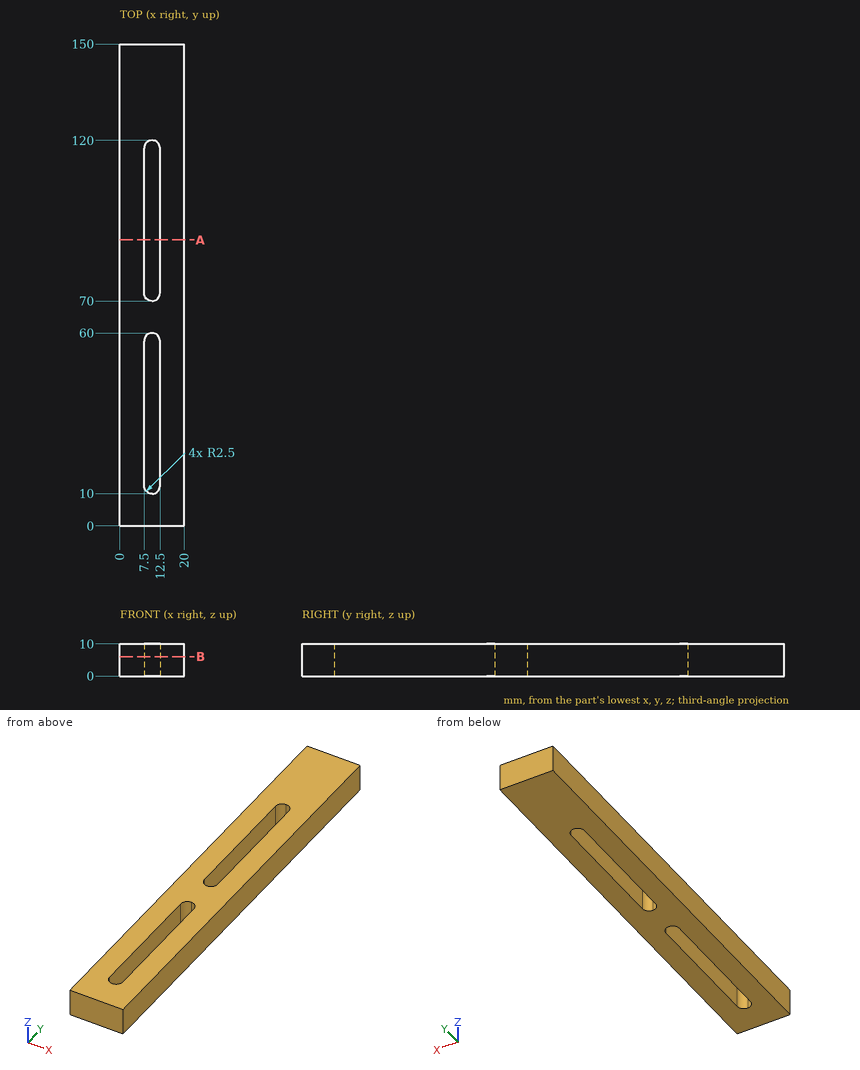
Geometry check sheet. Reference: drawing and pictorial views, mm from the part's lowest x, y, z. Give positions to 0.01 mm unless a question says otherwise; leave off trailing zeros. Write each loop counter-clockwise with the first axis right and the second up, starting at its lowest first coordinate (ties: lowest second). Pieces come first, ordered by that corner, then holes. Notation, with made-up numbers: M 21,22.25 L 54,22.25 A14 cw 54,30.25 Z; hole C 75,37 d1. An arc over 180 degrees is marked long. Put each result on its own line as item: value. Start each with the question number.
1. Scan line: line 1 along X through (y, z) = (72.5, 7). Record every from-to range of solid material in increasing order. Write a range as [from, to].
2. Section check A-A (y = 89). Record the cut outline in (x, z), and give its area (3 significant figures).
3. Section check B-B (z = 6). Give the number of separate pieces and of enclosed holes in the cut face, and give its area (3 significant figures).
Answer list:
1. line 1: [0, 7.5], [12.5, 20]
2. outline: M 0,0 L 7.5,0 L 7.5,10 L 0,10 Z; M 12.5,0 L 20,0 L 20,10 L 12.5,10 Z
2. area: 150 mm2
3. separate pieces: 1
3. enclosed holes: 2
3. area: 2,510 mm2
